Work out the finished part from the listing and answer in its coordinate system (mm). Give positions to 0.01 mm unless a question says otherwise; leave off trailing zeros. Loops run counter-clockwise (first coordinate to the right, second up) from the corner with the lowest first, then second, coordinate; pieces in that order, holes last. Notation, with made-up numbers: (80.5, -10) - (137.5, -10) arc R30 ccw to (137.5, 20) - close; hole circle Ø1 at (9.5, 15). An arc over 180 degrees is marked (long way). One line per item, written item: value.
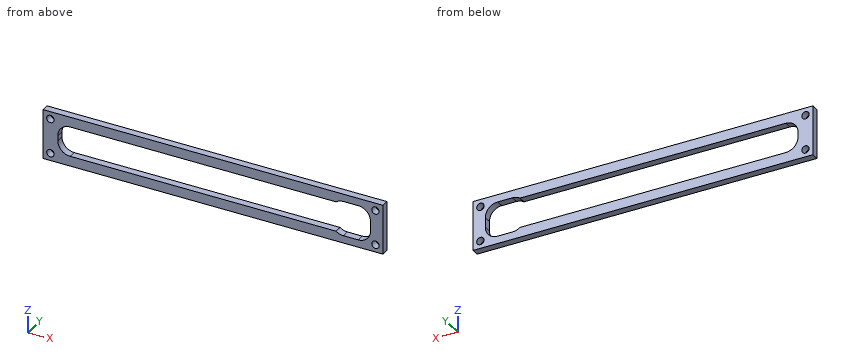
from build123d import *

# Parameters (mm, degrees)
SKETCH1_W           = 137.727780531
SKETCH1_H           = 20
SKETCH1_R           = 1.5
SKETCH1_W_2         = 125.727780531
SKETCH1_H_2         = 12
BOSS_EXTRUDE1_DEPTH = 3
CUT_EXTRUDE1_DEPTH  = 140.204674958
FILLET1_R           = 5


with BuildPart() as part:
    # Sketch1 → Boss-Extrude1 (new body)
    with BuildSketch(Plane(origin=(0, 0, 0), x_dir=(1, 0, 0), z_dir=(0, 1, 0))):
        with Locations((68.863890266, 10)):
            Rectangle(SKETCH1_W, SKETCH1_H)
        with Locations(Location((3, 17, 0), (0, 0, 270))):
            Circle(SKETCH1_R, mode=Mode.SUBTRACT)
        with Locations(Location((3, 3, 0), (0, 0, 90))):
            Circle(SKETCH1_R, mode=Mode.SUBTRACT)
        with Locations(Location((134.727780531, 3, 0), (0, 0, 270))):
            Circle(SKETCH1_R, mode=Mode.SUBTRACT)
        with Locations(Location((134.727780531, 17, 0), (0, 0, 90))):
            Circle(SKETCH1_R, mode=Mode.SUBTRACT)
        with Locations((68.863890266, 10)):
            Rectangle(SKETCH1_W_2, SKETCH1_H_2, mode=Mode.SUBTRACT)
    extrude(amount=BOSS_EXTRUDE1_DEPTH)

    # Sketch2 → Cut-Extrude1 (cut, through all)
    with BuildSketch(Plane(origin=(0, 3, 0), x_dir=(1, 0, 0), z_dir=(0, 1, 0))):
        Polygon((118.727780531, 17), (118.727780531, 16), (131.727780531, 16), (131.727780531, 4), (118.727780531, 4), (118.727780531, 3), (132.727780531, 3), (132.727780531, 17), align=None)
    extrude(amount=-CUT_EXTRUDE1_DEPTH, mode=Mode.SUBTRACT)

    # Fillet1
    # the kernel refuses this fillet: 5 mm, written as the material it adds along each edge
    with BuildSketch(Plane(origin=(132.727780531, 3, -17), x_dir=(0, 0, 1), z_dir=(0, -1, 0)), Plane(origin=(132.727780531, 3, -3), x_dir=(-1, 0, 0), z_dir=(0, -1, 0)), Plane(origin=(6, 0, -16), x_dir=(0, 0, 1), z_dir=(0, 1, 0))) as fillet1_piece_1:
        with BuildLine():
            CenterArc((FILLET1_R, FILLET1_R), FILLET1_R, 180, 90)
            Line((0, FILLET1_R), (-FILLET1_R * 0.02, FILLET1_R))
            Line((-FILLET1_R * 0.02, FILLET1_R), (-FILLET1_R * 0.02, -FILLET1_R * 0.02))
            Line((-FILLET1_R * 0.02, -FILLET1_R * 0.02), (FILLET1_R, -FILLET1_R * 0.02))
            Line((FILLET1_R, -FILLET1_R * 0.02), (FILLET1_R, 0))
        make_face()
    extrude(amount=3)
    with BuildSketch(Plane(origin=(118.727780531, 3, -17), x_dir=(1, 0, 0), z_dir=(0, -1, 0))) as fillet1_piece_2:
        with BuildLine():
            CenterArc((3, 5), FILLET1_R, 233.130102354, 36.869897646)
            Line((0, 1), (-0.06, 0.92))
            ThreePointArc((-0.06, 0.92), (-0.1, 0.5), (-0.1, 0))
            Line((-0.1, 0), (0, -0.1))
            Line((0, -0.1), (3, -0.1))
            Line((3, -0.1), (3, 0))
        make_face()
    extrude(amount=3)
    with BuildSketch(Plane(origin=(118.727780531, 3, -3), x_dir=(0, 0, -1), z_dir=(0, -1, 0))) as fillet1_piece_3:
        with BuildLine():
            CenterArc((5, 3), FILLET1_R, 180, 36.869897646)
            Line((0, 3), (-0.1, 3))
            Line((-0.1, 3), (-0.1, 0))
            Line((-0.1, 0), (0, -0.1))
            ThreePointArc((0, -0.1), (0.5, -0.1), (0.92, -0.06))
            Line((0.92, -0.06), (1, 0))
        make_face()
    extrude(amount=3)
    with BuildSketch(Plane(origin=(6, 0, -4), x_dir=(0, 0, -1), z_dir=(0, 1, 0))) as fillet1_piece_4:
        with BuildLine():
            CenterArc((FILLET1_R, -FILLET1_R), FILLET1_R, 90, 90)
            Line((0, -FILLET1_R), (-FILLET1_R * 0.02, -FILLET1_R))
            Line((-FILLET1_R * 0.02, -FILLET1_R), (-FILLET1_R * 0.02, FILLET1_R * 0.02))
            Line((-FILLET1_R * 0.02, FILLET1_R * 0.02), (FILLET1_R, FILLET1_R * 0.02))
            Line((FILLET1_R, FILLET1_R * 0.02), (FILLET1_R, 0))
        make_face()
    extrude(amount=3)


solid = part.part
1. Section C-C (y = 1.6) is taken. Write down the section's boundary in (x, z).
Output:
outline: (0, -20) - (137.73, -20) - (137.73, 0) - (0, 0) - close; hole circle Ø3 at (3, -17); hole circle Ø3 at (3, -3); hole (6, -11) arc R5 ccw to (11, -16) - (118.73, -16) arc R5 ccw to (121.73, -17) - (127.73, -17) arc R5 ccw to (132.73, -12) - (132.73, -8) arc R5 ccw to (127.73, -3) - (121.73, -3) arc R5 ccw to (118.73, -4) - (11, -4) arc R5 ccw to (6, -9) - close; hole circle Ø3 at (134.73, -17); hole circle Ø3 at (134.73, -3)
2. Find the intervals of material crossed by line 1 along Z through (x, y) = (34, 1.8); line 2 along X through (y, z) = (0.45, -1.75); line 3 along X through (y, z) = (1.65, -8.5), in increasing order.
Output:
line 1: z = -20 to -16, -4 to 0
line 2: x = 0 to 2.17, 3.83 to 133.9, 135.56 to 137.73
line 3: x = 0 to 6.03, 132.73 to 137.73
3. Section B-B (x = 3) is taken. Write down the section's boundary in (y, z), and give its area (3 significant figures).
Output:
outline: (0, -20) - (3, -20) - (3, -18.5) - (0, -18.5) - close; (0, -15.5) - (3, -15.5) - (3, -4.5) - (0, -4.5) - close; (0, -1.5) - (3, -1.5) - (3, 0) - (0, 0) - close
area: 42.0 mm²
4. Section A-A (x = 21.5) is taken. Write down the section's boundary in (y, z), and give its area (3 significant figures).
Output:
outline: (0, -20) - (3, -20) - (3, -16) - (0, -16) - close; (0, -4) - (3, -4) - (3, 0) - (0, 0) - close
area: 24.0 mm²
